Geometry check sheet. Reference: the model listing, model coordinates, mm. Face numbers are marked on the shaded views. Give positions to 0.01 mm unless a question says otherwise; leave off trailing zeros. Order: outer loops, then holes, each group sorted by start corner. A loop starts at its lowest first (then second) coordinate and runs counter-clockwise, first axis right, second up. Notation, with made-up numbers: M 77.5,-28.75 L 93.5,-28.75 A15 ccw 93.5,-11.75 Z; hole C 10.25,40 d1. An arc over 180 degrees is marked long. Put each result on its own line as item: value. Start each with the question number.
Q1. Section check B-B on y = 27.5. Record the cut outline in (x, z), then the cut area to 3 significant figures.
Q2. Section check A-A on x = 50. Record the cut outline in (y, z), then the cut area to 3 significant figures.
Q3. Go/stop test with a flat-tipped pin: pin 1 (11 mm diameter, centred on x = 50, z = -60, fed in from -Y). Record where the tip stops, or that it passes through.
Q4. Mould release check, pull along Z, two halves, no side actions. Record for the marked faces 1, 2 and 3: +Z half, -Z half, draft (parallel to the pull), parting line (faces both ways), or undercut.
Q5. Material ranges on L1, parallel to X at y = 1.45, z = -60; L2, parallel to Y at x = 265, z = -44; L3, parallel to Z at x = 50, y = 1.9, recorded low to high.
Q6. Section check D-D on z = -33. Record the cut outline in (x, y), then the cut area to 3 significant figures.
Q7. Section check C-C on z = -60. Record the cut outline in (x, y), then the cut area to 3 significant figures.
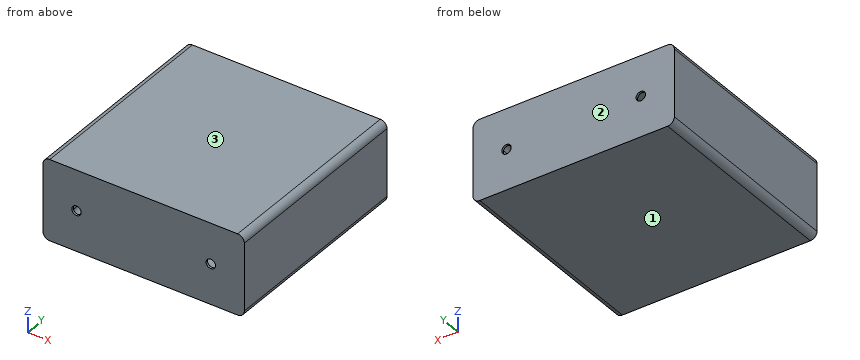
```python
from build123d import *

# Parameters (mm, degrees)
BOSS_EXTRUDE1_DEPTH     = 300
SHELL5_T                = -3
BOSS_EXTRUDE2_DEPTH     = 3
CUT_EXTRUDE1_DEPTH      = 443.954850972
CUT_EXTRUDE1_DEPTH_BACK = 443.954850972
SKETCH4_R               = 7


with BuildPart() as part:
    # Sketch2 → Boss-Extrude1 (new body)
    with BuildSketch(Plane(origin=(0, 0, 0), x_dir=(1, 0, 0), z_dir=(0, 1, 0))):
        with BuildLine():
            Line((10, 0), (290, 0))
            ThreePointArc((290, 0), (297.071067812, 2.928932188), (300, 10))
            Line((300, 10), (300, 110))
            ThreePointArc((300, 110), (297.071067812, 117.071067812), (290, 120))
            Line((290, 120), (10, 120))
            ThreePointArc((10, 120), (2.928932188, 117.071067812), (0, 110))
            Line((0, 110), (0, 10))
            ThreePointArc((0, 10), (2.928932188, 2.928932188), (10, 0))
        make_face()
    extrude(amount=BOSS_EXTRUDE1_DEPTH)

    # Shell5
    shell5_openings = [part.faces().sort_by_distance(p)[0] for p in [
        (150, 300, -60),
    ]]
    offset(amount=SHELL5_T, openings=shell5_openings, kind=Kind.INTERSECTION)

    # Sketch3 → Boss-Extrude2 (add)
    with BuildSketch(Plane(origin=(0, 300, 0), x_dir=(1, 0, 0), z_dir=(0, 1, 0))):
        with BuildLine():
            Line((10, 0), (290, 0))
            ThreePointArc((290, 0), (297.071067812, 2.928932188), (300, 10))
            Line((300, 10), (300, 110))
            ThreePointArc((300, 110), (297.071067812, 117.071067812), (290, 120))
            Line((290, 120), (10, 120))
            ThreePointArc((10, 120), (2.928932188, 117.071067812), (0, 110))
            Line((0, 110), (0, 10))
            ThreePointArc((0, 10), (2.928932188, 2.928932188), (10, 0))
        make_face()
    extrude(amount=BOSS_EXTRUDE2_DEPTH)

    # Sketch4 → Cut-Extrude1 (cut, two sides: drawn at the far end of the back side and taken through both)
    with BuildSketch(Plane(origin=(0, 303, 0), x_dir=(1, 0, 0), z_dir=(0, 1, 0)).offset(-CUT_EXTRUDE1_DEPTH_BACK)):
        with Locations(Location((50, 60, 0), (0, 0, 270))):
            Circle(SKETCH4_R)
        with Locations(Location((250, 60, 0), (0, 0, 270))):
            Circle(SKETCH4_R)
    extrude(amount=CUT_EXTRUDE1_DEPTH + CUT_EXTRUDE1_DEPTH_BACK, mode=Mode.SUBTRACT)


solid = part.part
```
Results found:
1. outline: M 0,-110 A10 ccw 10,-120 L 290,-120 A10 ccw 300,-110 L 300,-10 A10 ccw 290,0 L 10,0 A10 ccw 0,-10 Z; hole M 3,-110 A7 ccw 10,-117 L 290,-117 A7 ccw 297,-110 L 297,-10 A7 ccw 290,-3 L 10,-3 A7 ccw 3,-10 Z
1. area: 2,440 mm^2
2. outline: M 0,-120 L 303,-120 L 303,-67 L 300,-67 L 300,-117 L 3,-117 L 3,-67 L 0,-67 Z; M 0,-53 L 3,-53 L 3,-3 L 300,-3 L 300,-53 L 303,-53 L 303,0 L 0,0 Z
2. area: 2,420 mm^2
3. pin 1: passes through
4. face 1: -Z half
4. face 2: draft
4. face 3: +Z half
5. L1: x = 0 to 43, 57 to 243, 257 to 300
5. L2: y = 0 to 3, 300 to 303
5. L3: z = -120 to -67, -53 to 0
6. outline: M 0,0 L 300,0 L 300,303 L 0,303 Z; hole M 3,3 L 297,3 L 297,300 L 3,300 Z
6. area: 3,580 mm^2
7. outline: M 0,0 L 43,0 L 43,3 L 3,3 L 3,300 L 43,300 L 43,303 L 0,303 Z; M 57,0 L 243,0 L 243,3 L 57,3 Z; M 57,300 L 243,300 L 243,303 L 57,303 Z; M 257,0 L 300,0 L 300,303 L 257,303 L 257,300 L 297,300 L 297,3 L 257,3 Z
7. area: 3,410 mm^2
